Work out the finished part from the listing and answer in its coordinate system (mm). A direction names the side the tool comes from. Coordinates: 2 decimals unless noted, no trailing zeros. Order: outer loops, then holes, each group sorted by start corner. A loop starts at its lowest first (then second) coordinate and runs counter-clockwise, first axis right, second up. Notation, with made-up numbers: (-6, 21) -> (22, 21) arc R19 ccw to (22, 27) -> close; hole circle Ø4 at (74, 34). An arc over 180 degrees is marked (long way). Answer as CSV lines item,"result". Start each with the question number.
Item 1: Straight lines are drawn through the part: L1, parallel to Y at x = -3, z = 3.2; L2, parallel to Y at x = -3.5, z = 4.6; L3, parallel to Y at x = -31.5, z = 4.1. For each, find the intervals that lie inside material, in ascending order.
Item 2: Which of the six approach directions +Z, -Z, +X, -X, +Y, -Y give full straight-line access (tool end or side, diameter ignored) to faces 5 (the face through (-1, 24.9, 3)), 6 (the face through (0, 3, 3)), 7 (the face through (-35, 18, 3))?
Item 3: For a pull along Y with two mould halves and no side action, classify faces 1 (the face through (-42, 8, 3)), 2 (the face through (-26, 31.3, 3)), 3 (the face through (-36, 24.9, 3)), 4 (the face through (-39, 4.5, 3)) as pulls with the +Y half, pulls with the -Y half, needs draft (parallel to the pull), parting line crosses it, or undercut.
Item 4: Section A-A (z = 4.9) is taken. Write down the section's boundary in (x, y).
Item 5: Each of these flat-tipped pins is pushed along its axis until it touches: pin 1 Ø1.8 at (x, z) = (1, 2.5) entering from +Y; pin 2 Ø1 at (x, z) = (-36, 3.5) entering from -Y; pin 3 Ø1.3 at (y, z) = (27, 1.5) entering from -X; pin 4 Ø2.5 at (x, y) = (-3, 34) entering from +Z. Where does it stop, or does it pass through?
Item 6: Section B-B (y = 34) is taken. Write down the section's boundary in (x, z), then the cut area to 3 significant figures.
Item 7: Section D-D (x = -3) is taken. Write down the section's boundary in (y, z).
Item 8: Section C-C (x = -31.5) is taken. Write down the section's boundary in (y, z).
Autodesk Inventor part; units mm, degrees
ref_plane "YZ Plane" through (0, 0, 0) normal (1, 0, 0) x (0, 1, 0)
ref_plane "XZ Plane" through (0, 0, 0) normal (0, 1, 0) x (-1, 0, 0)
ref_plane "XY Plane" through (0, 0, 0) normal (0, 0, 1) x (1, 0, 0)
sketch "Sketch1" plane through (0, 0, 0) normal (0, 0, 1) x (1, 0, 0)
  arc A0 (-2, 0) -> (0, 2) centre (-2, 2) ccw
  line L0 (0, 4.5) -> (0, 2)
  line L1 (5, 4.5) -> (0, 4.5)
  line L2 (5, 10.9) -> (5, 4.5)
  line L3 (-2, 10.9) -> (5, 10.9)
  line L4 (-2, 24.9) -> (-2, 10.9)
  line L5 (0, 24.9) -> (-2, 24.9)
  line L6 (0, 35) -> (0, 24.9)
  arc A1 (0, 35) -> (-2, 37) centre (-2, 35) ccw
  line L7 (-13, 37) -> (-2, 37)
  arc A2 (-13, 37) -> (-15, 35) centre (-13, 35) ccw
  line L8 (-15, 33.3) -> (-15, 35)
  arc A3 (-17, 31.3) -> (-15, 33.3) centre (-17, 33.3) ccw
  line L9 (-35, 31.3) -> (-17, 31.3)
  arc A4 (-35, 31.3) -> (-37, 29.3) centre (-35, 29.3) ccw
  line L10 (-37, 24.9) -> (-37, 29.3)
  line L11 (-35, 24.9) -> (-37, 24.9)
  line L12 (-35, 10.9) -> (-35, 24.9)
  line L13 (-42, 10.9) -> (-35, 10.9)
  line L14 (-42, 4.5) -> (-42, 10.9)
  line L15 (-37, 4.5) -> (-42, 4.5)
  line L16 (-37, 2) -> (-37, 4.5)
  arc A5 (-37, 2) -> (-35, 0) centre (-35, 2) ccw
  line L17 (-2, 0) -> (-35, 0)
  circle A6 centre (-3, 34) radius 1.5
  circle A7 centre (-34, 3) radius 1.5
  circle A8 centre (-3, 3) radius 1.5
  circle A9 centre (-31.5, 26.9) radius 1.5
  point P0 (0, 0)
  point P1 (0, 0)
extrude "Extrusion1" add sketch "Sketch1" along normal blind 6
properties part number "XcrRightTop"
Checked values:
1,L1,"y = 0 to 1.5, 4.5 to 32.5, 35.5 to 37"
1,L2,"y = 0 to 1.59, 4.41 to 32.59, 35.41 to 37"
1,L3,"y = 0 to 25.4, 28.4 to 31.3"
2,face 5,"+Z, -Z, +X"
2,face 6,"+Z, -Z, +X, -Y"
2,face 7,"+Z, -Z, -X"
3,face 1,"needs draft"
3,face 2,"pulls with the +Y half"
3,face 3,"undercut"
3,face 4,"pulls with the -Y half"
4,outline,"(-42, 4.5) -> (-37, 4.5) -> (-37, 2) arc R2 ccw to (-35, 0) -> (-2, 0) arc R2 ccw to (0, 2) -> (0, 4.5) -> (5, 4.5) -> (5, 10.9) -> (-2, 10.9) -> (-2, 24.9) -> (0, 24.9) -> (0, 35) arc R2 ccw to (-2, 37) -> (-13, 37) arc R2 ccw to (-15, 35) -> (-15, 33.3) arc R2 cw to (-17, 31.3) -> (-35, 31.3) arc R2 ccw to (-37, 29.3) -> (-37, 24.9) -> (-35, 24.9) -> (-35, 10.9) -> (-42, 10.9) -> close; hole circle Ø3 at (-34, 3); hole circle Ø3 at (-31.5, 26.9); hole circle Ø3 at (-3, 3); hole circle Ø3 at (-3, 34)"
5,pin 1,"stops at y = 10.9"
5,pin 2,"stops at y = 0.06"
5,pin 3,"stops at x = -37"
5,pin 4,"passes through"
6,outline,"(-15, 0) -> (-4.5, 0) -> (-4.5, 6) -> (-15, 6) -> close; (-1.5, 0) -> (0, 0) -> (0, 6) -> (-1.5, 6) -> close"
6,area,"72.0 mm^2"
7,outline,"(0, 0) -> (1.5, 0) -> (1.5, 6) -> (0, 6) -> close; (4.5, 0) -> (32.5, 0) -> (32.5, 6) -> (4.5, 6) -> close; (35.5, 0) -> (37, 0) -> (37, 6) -> (35.5, 6) -> close"
8,outline,"(0, 0) -> (25.4, 0) -> (25.4, 6) -> (0, 6) -> close; (28.4, 0) -> (31.3, 0) -> (31.3, 6) -> (28.4, 6) -> close"
